Verification items for the finished model (mm, model axes). Give positions to 0.01 mm unless a question says otherwise; leave off trailing zeros. Write each loop counter-clockwise with the first axis right and the second up, starting at its lowest first coordinate (ties: lowest second). Pieces come first, ordered by that corner, then holes. Notation, with made-up numbers: (-15.75, -6.75) - (33.25, -6.75) arc R29 ccw to (33.25, 21.25) - close; hole circle Ø6 at (31.25, -28). An arc over 180 degrees is marked (long way). Put each result on its own line as item: value.
Autodesk Inventor part; units mm, degrees
ref_plane "YZ Plane" through (0, 0, 0) normal (1, 0, 0) x (0, 1, 0)
ref_plane "XZ Plane" through (0, 0, 0) normal (0, 1, 0) x (-1, 0, 0)
ref_plane "XY Plane" through (0, 0, 0) normal (0, 0, 1) x (1, 0, 0)
sketch "Sketch1" plane through (0, 0, 0) normal (0, 0, 1) x (1, 0, 0)
  circle A0 centre (0, 0) radius 1.5875
  line L0 (-4.6927, 0) -> (-2.3464, 4.064)
  line L1 (-2.3464, 4.064) -> (2.3464, 4.064)
  line L2 (2.3464, 4.064) -> (4.6927, 0)
  line L3 (4.6927, 0) -> (2.3464, -4.064)
  line L4 (2.3464, -4.064) -> (-2.3464, -4.064)
  line L5 (-2.3464, -4.064) -> (-4.6927, 0)
  dimension "d0" = 3.175
  dimension "d1" = 8.128
extrude "Extrusion1" add sketch "Sketch1" along normal blind 7.112
sketch "Sketch2" plane through (2.3464, 4.064, 7.112) normal (0.866, 0.5, 0) x (0, 0, -1)
  circle A0 centre (3.556, -2.3464) radius 1.27
  line L0 (0, -4.6927) -> (0, 0)
  line L1 (7.112, 0) -> (7.112, -4.6927)
  line L2 (7.112, 0) -> (0, 0)
  line L3 (0, -4.6927) -> (0, 0)
  line L4 (7.112, -4.6927) -> (0, -4.6927)
  line L5 (3.556, -2.3464) -> (3.556, 0) construction
  line L6 (7.112, 0) -> (0, 0) construction
  line L7 (3.556, -2.3464) -> (3.556, -4.6927) construction
  line L8 (7.112, -4.6927) -> (0, -4.6927) construction
  line L9 (3.556, -2.3464) -> (0, -2.3464) construction
  line L10 (3.556, -2.3464) -> (7.112, -2.3464) construction
  line L11 (7.112, -4.6927) -> (7.112, 0) construction
  dimension "d4" = 2.54
extrude "Extrusion2" cut sketch "Sketch2" against normal up to next contours A0
properties part number ".125InchShaftHexNut" material "Brass, Soft Yellow"
Q1. Section check C-C, the plane y = -0.75. Record the cut outline in (x, z), plus the area to 3 significant figures.
Answers follow:
outline: (-4.26, 0) - (-1.4, 0) - (-1.4, 7.11) - (-4.26, 7.11) - close; (1.4, 0) - (4.26, 0) - (4.26, 7.11) - (1.4, 7.11) - close
area: 40.7 mm2
Q2. Scan lines: line 1 along Y through (x, z) = (0, 1.5); line 2 along Z through (x, y) = (3, 1); line 3 along Y through (x, z) = (-2.5, 6). Record each from-to range of solid material in increasing order.
Answers follow:
line 1: y = -4.06 to -1.59, 1.59 to 4.06
line 2: z = 0 to 2.46, 4.66 to 7.11
line 3: y = -3.8 to 3.8
Q3. Go/stop test with flat-tipped pins: pin 1 Ø2 at (y, z) = (-2, 1.5) entering from +X; pin 2 Ø1 at (y, z) = (-2.5, 4) entering from +X; pin 3 Ø2 at (x, z) = (-3.5, 3.5) entering from +Y. Record where each tip stops, or that it passes through.
Answers follow:
pin 1: stops at x = 4.12
pin 2: stops at x = 3.54
pin 3: stops at y = 3.8
Q4. Section check B-B, the plane x = 0. Record the cut outline in (y, z).
Answers follow:
outline: (-4.06, 0) - (-1.59, 0) - (-1.59, 7.11) - (-4.06, 7.11) - close; (1.59, 0) - (4.06, 0) - (4.06, 7.11) - (1.59, 7.11) - close
Q5. Section check D-D, the plane z = 4.25. Record the cut outline in (x, y) (1 decimal).
Answers follow:
outline: (-4.7, 0) - (-2.3, -4.1) - (2.3, -4.1) - (4.7, 0) - (4.1, 1.1) - (1.6, -0.3) arc R1.6 cw (long way) to (0.5, 1.5) - (3, 3) - (2.3, 4.1) - (-2.3, 4.1) - close
Q6. Section check A-A, the plane z = 5. Record the cut outline in (x, y) (1 decimal).
Answers follow:
outline: (-4.7, 0) - (-2.3, -4.1) - (2.3, -4.1) - (4.7, 0) - (2.3, 4.1) - (-2.3, 4.1) - close; hole circle Ø3.2 at (0, 0)
Q7. Release check for a two-part mould opening along X. For faces 1 (the face through (0, -4.064, 4)), 2 (the face through (2.577, 0.596, 4.564)), 3 (the face through (-3.503, -2.06, 3.506)) record: released by +X, released by -X, zero draft, split by the parting line, or undercut.
Answers follow:
face 1: zero draft
face 2: undercut
face 3: released by -X
